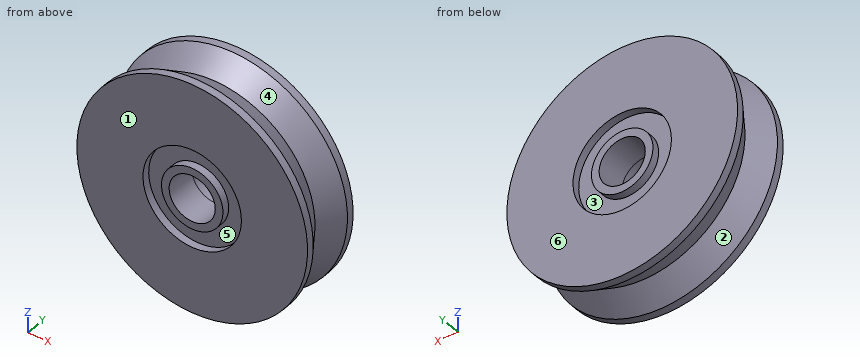
from build123d import *


with BuildPart() as part:
    # Sketch1 → Revolve1 (revolve)
    with BuildSketch(Plane.XY, mode=Mode.PRIVATE) as revolve1_sk:
        Polygon((-1.5, 0), (-1.5, 2), (-2, 2), (-2, 1.5), (-3.2, 1.5), (-3.2, 2), (-7.5, 2), (-7.5, 1.5), (-6.5, 0), align=None)
    revolve1 = revolve(revolve1_sk.sketch.rotate(Axis((0, 0, 0), (0, 1, 0)), 270), axis=Axis((0, 0, 0), (0, 1, 0)))

    # Mirror1: Revolve1 across plane
    add(revolve1.mirror(Plane(origin=(-6.5, 0, 0), x_dir=(0, 0, 1), z_dir=(0, 1, 0))))


solid = part.part
The listing builds one solid part. Answer for the finished solid, in the listing's coordinates (mm). Face numbers are marked on the shaded views. A direction names the side the tool comes from. Give positions to 0.01 mm unless a question says otherwise; leave off trailing zeros. Write each loop counter-clockwise with the first axis right and the second up, starting at its lowest first coordinate (ties: lowest second). Pieces come first, ordered by that corner, then holes.
1) Section C-C (y = 0.95) is taken. Write down the section's boundary in (x, z), and give its area (3 significant figures).
2) Section D-D (y = -0.7) is taken. Write down the section's boundary in (x, z), and give its area (3 significant figures).
3) For a pull along X with two mould halves and no side action, classify the marked faces 1, 2 and 3 as pulls with the +X half, pulls with the -X half, needs draft (parallel to the pull), parting line crosses it, or undercut.
4) A tool of negligible diameter and unlimited length cuts with its end or side. For the marked faces 4, 5 and 6, from which of +Z, -Z, +X, -X, +Y, -Y can it reach the whole face along a straight path? Write none if from no direction.
5) Find the intervals of material crossed by L1, parallel to X at y = 1.65, z = 0; L2, parallel to X at y = 1.3, z = 0; L3, parallel to Y at x = 5, z = -5.5, in increasing order.
6) Given P1, Ø2.5, axis at x = 0, z = 0, coming from the +Y side; P2, Ø1.5, axis at x = 5, y = 0, coming from the -Z side; P3, Ø2, axis at x = -6, y = -0.5, coming from the -Z side, each flat-ended and moving along its own axis, determine where each tip first touches the part or whether it passes through.
Response:
1. outline: circle Ø14.27 at (0, 0); hole circle Ø3 at (0, 0)
1. area: 153 mm2
2. outline: circle Ø13.93 at (0, 0); hole circle Ø3 at (0, 0)
2. area: 145 mm2
3. face 1: needs draft
3. face 2: parting line crosses it
3. face 3: undercut
4. face 4: none
4. face 5: -Y
4. face 6: +Z, -Z, +X, -X, +Y
5. L1: x = -7.5 to -3.2, -2 to -1.5, 1.5 to 2, 3.2 to 7.5
5. L2: x = -7.37 to -1.5, 1.5 to 7.37
5. L3: y = -2 to -1.4, 1.4 to 2
6. P1: passes through
6. P2: stops at z = -5.2
6. P3: stops at z = -5.04
